```python
from build123d import *

# Parameters (mm, degrees)
SKETCH1_R           = 2.54
BOSS_EXTRUDE1_DEPTH = 2.54
SKETCH2_W           = 38.1
SKETCH2_H           = 38.1
SKETCH2_R           = 2.54
BOSS_EXTRUDE2_DEPTH = 2.54
FILLET2_R           = 2.54
FILLET3_R           = 2.54


with BuildPart() as part:
    # Sketch1 → Boss-Extrude1 (new body)
    with BuildSketch(Plane(origin=(0, 0, 0), x_dir=(1, 0, 0), z_dir=(0, 1, 0))):
        Polygon((-19.583364039, 14.230768135), (-5.08, 14.230768135), (5.08, 14.230768135), (18.516635961, 14.230768135), (18.516635961, -13.709231865), (-19.583364039, -13.709231865), align=None)
        with Locations(Location((-11.201364039, -1.009231865, 0), (0, 0, 270))):
            Circle(SKETCH1_R, mode=Mode.SUBTRACT)
        with Locations(Location((10.134635961, -1.009231865, 0), (0, 0, 270))):
            Circle(SKETCH1_R, mode=Mode.SUBTRACT)
    extrude(amount=BOSS_EXTRUDE1_DEPTH)

    # Sketch2 → Boss-Extrude2 (add)
    with BuildSketch(Plane.XY.offset(13.709231865)):
        with Locations((-0.533364039, -16.51)):
            Rectangle(SKETCH2_W, SKETCH2_H)
        with Locations((-0.533364039, -12.7)):
            Circle(SKETCH2_R, mode=Mode.SUBTRACT)
        with Locations((-0.533364039, -26.67)):
            Circle(SKETCH2_R, mode=Mode.SUBTRACT)
    extrude(amount=BOSS_EXTRUDE2_DEPTH)

    # Fillet2
    fillet2_edges = [part.edges().sort_by_distance(p)[0] for p in [
        (-0.533364039, 0, 13.709231865),
    ]]
    fillet(fillet2_edges, radius=FILLET2_R)

    # Fillet3
    fillet3_edges = [part.edges().sort_by_distance(p)[0] for p in [
        (-0.533364039, 2.54, 16.249231865),
    ]]
    fillet(fillet3_edges, radius=FILLET3_R)


solid = part.part
```
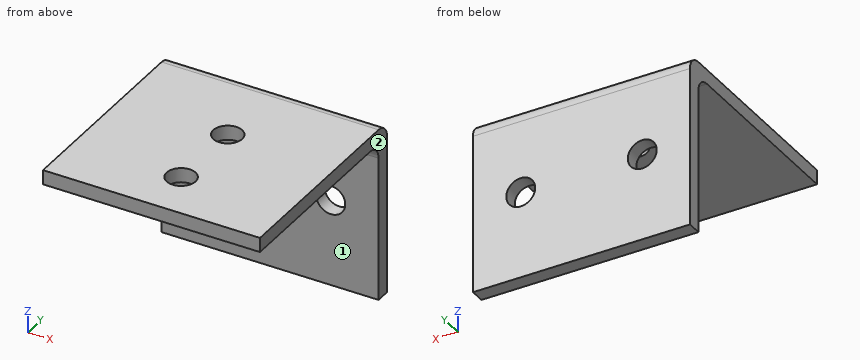
The model under review builds one solid part; all positions refer to its coordinate system, in mm. Face numbers are marked on the shaded views. A direction names the side the tool comes from. Round coordinates to 2 decimals unless told otherwise and drop trailing zeros. Write each loop counter-clockwise with the first axis right and the second up, starting at its lowest first coordinate (ties: lowest second). Pieces come first, ordered by that corner, then holes. Notation, with made-up numbers: (15.5, 63.5) - (45.5, 63.5) arc R34 cw to (45.5, 95.5) - close; hole circle Ø4 at (20, -30). An arc over 180 degrees is marked (long way). Use one line per item in the form item = value.
Q1. For line 1 (Y direction, x = 16.5, z = -12); line 2 (Z direction, x = 10, y = -26); line 3 (Y direction, x = 4.5, z = 12.5), list the stretches that pass through material, from the lowest coordinate up. Write a range as [from, to].
Answer key:
line_1 = [0, 2.54]
line_2 = [13.71, 16.25]
line_3 = [-0.38, 2.54]
Q2. Tool access review of the marked faces 1 and 2: name each direction out of +Z, -Z, +X, -X, +Y, -Y from which nothing blocks a thin tool from reaching the whole face with its end or side.
Answer key:
face_1 = -Z, +X, -X, -Y
face_2 = +Z, -Z, +X, +Y, -Y
Q3. Consider section A-A (y = -26.67). State the section outline as (x, z) points, and give its area (3 significant figures).
Answer key:
outline = (-19.58, 13.71) - (-3.07, 13.71) - (-3.07, 16.25) - (-19.58, 16.25) - close; (2.01, 13.71) - (18.52, 13.71) - (18.52, 16.25) - (2.01, 16.25) - close
area = 83.9 mm2
Q4. Consider section D-D (y = -22). State the section outline as (x, z) points.
Answer key:
outline = (-19.58, 13.71) - (18.52, 13.71) - (18.52, 16.25) - (-19.58, 16.25) - close
Q5. Consider section C-C (x = 12). State the section outline as (y, z) points.
Answer key:
outline = (-35.56, 13.71) - (-2.54, 13.71) arc R2.54 cw to (0, 11.17) - (0, 2.73) - (2.54, 2.73) - (2.54, 13.71) arc R2.54 ccw to (0, 16.25) - (-35.56, 16.25) - close; (0, -14.23) - (2.54, -14.23) - (2.54, -0.71) - (0, -0.71) - close
Q6. Consider section B-B (x = -1). State the section outline as (y, z) points, and give its area (3 significant figures).
Answer key:
outline = (-35.56, 13.71) - (-29.17, 13.71) - (-29.17, 16.25) - (-35.56, 16.25) - close; (-24.17, 13.71) - (-15.2, 13.71) - (-15.2, 16.25) - (-24.17, 16.25) - close; (-10.2, 13.71) - (-2.54, 13.71) arc R2.54 cw to (0, 11.17) - (0, -14.23) - (2.54, -14.23) - (2.54, 13.71) arc R2.54 ccw to (0, 16.25) - (-10.2, 16.25) - close
area = 142 mm2
Q7. Insertion check: pin 1 Ø1.5 at (x, z) = (-6.5, -4) entering from -Y; pin 2 Ø1 at (x, y) = (3, -3) entering from -Z. Each pin has a flat end and moves straight along its axis. Give the tip position at first contact, or say it passes through.
Answer key:
pin_1 = 0
pin_2 = 13.71
